The model under review builds one solid part; all positions refer to its coordinate system, in mm. A direction names the side the tool comes from. Round coordinates to 2 decimals unless told otherwise and drop trailing zeros. Order: outer loops, then holes, each group sorted by start corner. A loop starts at its lowest first (then second) coordinate and runs counter-clockwise, first axis right, second up. Notation, with made-up numbers: M -11.5,69.5 L 21.5,69.5 A19 ccw 21.5,90.5 Z; hole C -36.75,7 d9. An arc over 180 degrees is marked long. Use a Markdown table: item, result. Add a question column.
1. Consider section C-C on z = 1.3. Count the separate pieces of the cut face and the enclosed holes in it, then the cut area to 3 significant figures.
2. To check wall thickness, follow probe 1 along Y at (x, z) = (0, 0.6); probe 2 along Y at (x, z) = (25, 1.3); probe 3 along X at (y, z) = (26.5, 1.5). State the ranges of each line that lie inside material, in increasing order.
3. The part is to be moulded in two halves that separate along X. For faces 5 (the cylindrical face through (31.359, 6.637, 1.479)), 6 (the flat face through (-32.5, -15, 1)), 7 (the cylindrical face through (-24.24, -39.75, 1.48)), say which applies: +X half, -X half, draft (parallel to the pull), parting line (faces both ways), or undercut.
4. For faces 1 (the flat face through (-16.25, 23, 2)), 2 (the flat face through (16.25, 23, 2)), 3 (the flat face through (-19.25, 34, 1)), 4 (the cylindrical face through (14.49, -17.12, 1.48)), list the 3-axis set-ups (+Z, -Z, +X, -X, +Y, -Y) from which the entire face can be reached by the end or side of a thin tool; tool diameter is ignored.
5. Insertion check: P1, Ø1.5, axis at y = 37.5, z = 1.5, coming from the +X side; P2, Ø1.5, axis at y = 37.5, z = 1.5, coming from the -X side; P3, Ø1.5, axis at x = 6.5, z = 1, coming from the +Y side. Each pin has a flat end and moves straight along its axis. Give the tip position at first contact, or say it passes through.
6. Consider section B-B on x = 0. State the section outline as (y, z) points, then the cut area to 3 significant figures.
7. Consider section A-A on y = -27. State the section outline as (x, z) points, then the cut area to 3 significant figures.
from build123d import *

# Parameters (mm, degrees)
SKETCH1_R           = 2.6
SKETCH1_R_2         = 10.25
BOSS_EXTRUDE1_DEPTH = 3
SKETCH2_W           = 3
SKETCH2_H           = 10
SKETCH2_W_2         = 10
SKETCH2_H_2         = 3
CUT_EXTRUDE1_DEPTH  = 3


with BuildPart() as part:
    # Sketch1 → Boss-Extrude1 (new body)
    with BuildSketch(Plane.XY):
        with BuildLine():
            Line((-32.5, -1.160301848), (-32.5, -34.265434942))
            ThreePointArc((-32.5, -34.265434942), (-24.085532921, -39.728848894), (-17.5, -32.160301848))
            Line((-17.5, -32.160301848), (-17.5, -24.27061763))
            ThreePointArc((-17.5, -24.27061763), (-14.571067812, -17.199549819), (-7.5, -14.27061763))
            Line((-7.5, -14.27061763), (7.5, -14.27061763))
            ThreePointArc((7.5, -14.27061763), (14.571067812, -17.199549819), (17.5, -24.27061763))
            Line((17.5, -24.27061763), (17.5, -32.160301848))
            Line((17.5, -32.160301848), (17.5, -36.245484302))
            ThreePointArc((17.5, -36.245484302), (25.631797985, -41.813464149), (32.5, -34.745484302))
            Line((32.5, -34.745484302), (32.5, -33.660301848))
            Line((32.5, -33.660301848), (32.5, -1.160301848))
            Line((32.5, -1.160301848), (32.5, 3.839698152))
            ThreePointArc((32.5, 3.839698152), (31.328427125, 6.668125276), (28.5, 7.839698152))
            Line((28.5, 7.839698152), (23.25, 7.839698152))
            ThreePointArc((23.25, 7.839698152), (20.421572875, 9.011271027), (19.25, 11.839698152))
            Line((19.25, 11.839698152), (19.25, 38.839698152))
            Line((19.25, 38.839698152), (-19.25, 38.839698152))
            Line((-19.25, 38.839698152), (-19.25, 11.839698152))
            ThreePointArc((-19.25, 11.839698152), (-20.421572875, 9.011271027), (-23.25, 7.839698152))
            Line((-23.25, 7.839698152), (-28.5, 7.839698152))
            ThreePointArc((-28.5, 7.839698152), (-31.328427125, 6.668125276), (-32.5, 3.839698152))
            Line((-32.5, 3.839698152), (-32.5, 3.273112401))
            Line((-32.5, 3.273112401), (-32.5, -1.160301848))
        make_face()
        with Locations((-25, -32.160301848)):
            Circle(SKETCH1_R, mode=Mode.SUBTRACT)
        with Locations((25, -32.160301848)):
            Circle(SKETCH1_R, mode=Mode.SUBTRACT)
        with Locations((0, 23.589698152)):
            Circle(SKETCH1_R_2, mode=Mode.SUBTRACT)
    extrude(amount=BOSS_EXTRUDE1_DEPTH)

    # Sketch2 → Cut-Extrude1 (cut)
    with BuildSketch(Plane.XY.offset(3)):
        with Locations((-17.75, 23.22062572)):
            Rectangle(SKETCH2_W, SKETCH2_H)
        with Locations((-8.827421787, 37.339698152)):
            Rectangle(SKETCH2_W_2, SKETCH2_H_2)
        with Locations((8.672578213, 37.339698152)):
            Rectangle(SKETCH2_W_2, SKETCH2_H_2)
        with Locations((17.75, 23.22062572)):
            Rectangle(SKETCH2_W, SKETCH2_H)
    extrude(amount=-CUT_EXTRUDE1_DEPTH, mode=Mode.SUBTRACT)


solid = part.part
Answer block:
| question | item | result |
|---|---|---|
| 1 | separate pieces | 1 |
| 1 | enclosed holes | 3 |
| 1 | area | 2,930 mm^2 |
| 2 | probe 1 | -14.27 to 13.34, 33.84 to 38.84 |
| 2 | probe 2 | -41.85 to -34.76, -29.56 to 7.84 |
| 2 | probe 3 | -16.25 to -9.83, 9.83 to 16.25 |
| 3 | face 5 | +X half |
| 3 | face 6 | -X half |
| 3 | face 7 | undercut |
| 4 | face 1 | +Z, -Z, -X |
| 4 | face 2 | +Z, -Z, +X |
| 4 | face 3 | +Z, -Z, -X, +Y |
| 4 | face 4 | +Z, -Z, -Y |
| 5 | P1 | x = 19.25 |
| 5 | P2 | x = -19.25 |
| 5 | P3 | y = 35.84 |
| 6 | outline | M -14.27,0 L 13.34,0 L 13.34,3 L -14.27,3 Z; M 33.84,0 L 38.84,0 L 38.84,3 L 33.84,3 Z |
| 6 | area | 97.8 mm^2 |
| 7 | outline | M -32.5,0 L -17.5,0 L -17.5,3 L -32.5,3 Z; M 17.5,0 L 32.5,0 L 32.5,3 L 17.5,3 Z |
| 7 | area | 90.0 mm^2 |
